Check sheet for the drawn part. Datum: minimum x, y, z corner. Units: mm. Give positions to 0.01 mm unless a question says otherwise; leave off trailing zeros. Order: outer loops, then holes, each group sorted by start corner. A loop starts at its lowest first (then second) coordinate and runs counter-clockwise, first axis right, second up. Notation, with made-up numbers: M 81.5,-7.75 L 126.5,-7.75 A13 ccw 126.5,9.25 Z; hole C -23,-30.5 d11. An arc over 180 degrees is marked long. Answer in a Markdown table with one row per item. Add a question column.
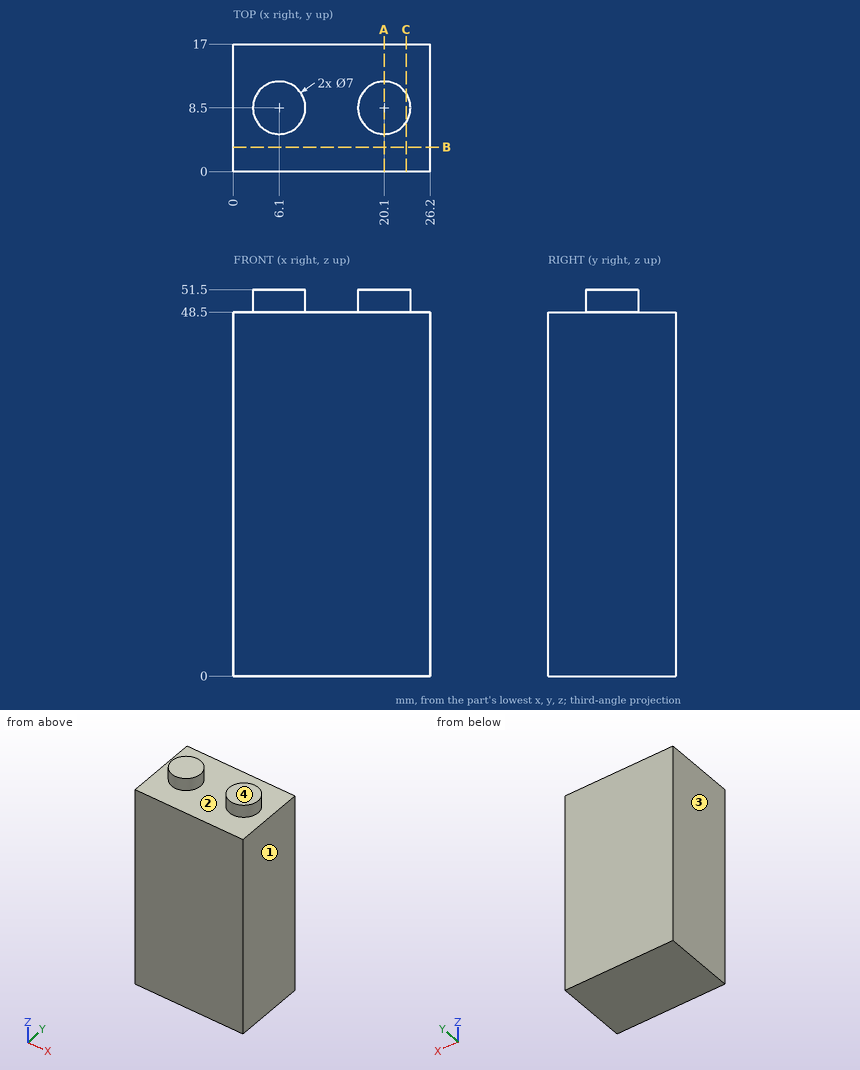
Q1. Draft check along X on the marked faces 1, 2, 3 and 4. Enter one of: pulls with the +X half, pulls with the -X half, needs draft (parallel to the pull), parting line crosses it, or undercut.
Q2. Thickness scan on probe 1 along Z at (x, y) = (19.25, 12.5). Record the ranges inside material, lowest first.
Q3. Cross-section at C-C (x = 23). Record the boundary of the cut face in (y, z), and give its area (3 significant figures).
Q4. Cross-section at A-A (x = 20.1). Record the boundary of the cut face in (y, z).
Q5. Cross-section at B-B (y = 3.25). Record the boundary of the cut face in (x, z), and give its area (3 significant figures).
Values follow:
| question | item | result |
|---|---|---|
| 1 | face 1 | pulls with the +X half |
| 1 | face 2 | undercut |
| 1 | face 3 | pulls with the -X half |
| 1 | face 4 | needs draft |
| 2 | probe 1 | 0 to 48.5 |
| 3 | outline | M 0,0 L 17,0 L 17,48.5 L 10.46,48.5 L 10.46,51.5 L 6.54,51.5 L 6.54,48.5 L 0,48.5 Z |
| 3 | area | 836 mm² |
| 4 | outline | M 0,0 L 17,0 L 17,48.5 L 12,48.5 L 12,51.5 L 5,51.5 L 5,48.5 L 0,48.5 Z |
| 5 | outline | M 0,0 L 26.2,0 L 26.2,48.5 L 0,48.5 Z |
| 5 | area | 1,270 mm² |
